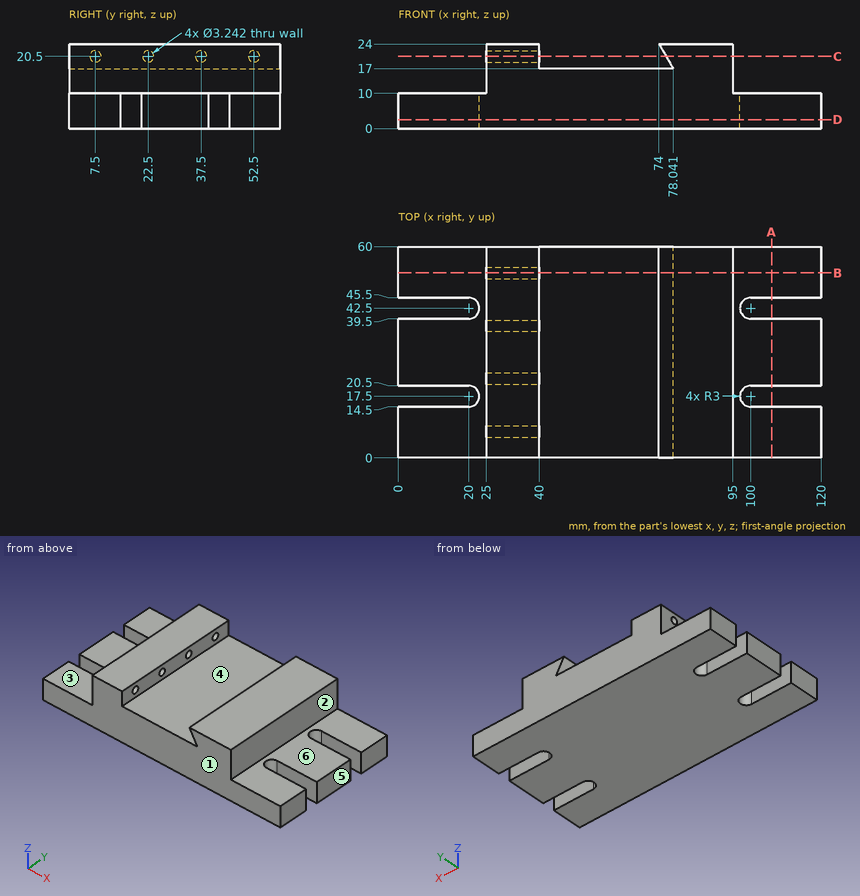
Geometry: see drawing. Coordinates: mm, zero at the bounding-box minimum. A direction names the side the tool comes from. Coordinates: 2 decimals unless noted, no trailing zeros. Order: outer loops, then holes, each group sorted by start corner. A loop starts at its lowest first (then second) coordinate and runs counter-clockwise, first axis right, second up. Notation, with made-up numbers: (-27, 75.25) - (2, 75.25) arc R21 ccw to (2, 102.25) - close; hole circle Ø3 at (63, 3). An arc over 180 degrees is marked (long way). Use one line per item in the form item = value.
1) Section A-A (x = 106). Return loops of the section in (y, z), then the cut area to 3 significant figures.
Solutions:
outline = (0, 0) - (14.5, 0) - (14.5, 10) - (0, 10) - close; (20.5, 0) - (39.5, 0) - (39.5, 10) - (20.5, 10) - close; (45.5, 0) - (60, 0) - (60, 10) - (45.5, 10) - close
area = 480 mm^2
2) Set-up query: the marked faces 1, 2 and 3. Return all of +Z, -Z, +X, -X, +Y, -Y with unobstructed straight access to the full face (end or side cutting, diameter ignored); none if empty.
Solutions:
face_1 = +Z, -Z, +X, -X, -Y
face_2 = +Z, +X, +Y, -Y
face_3 = +Z, -X, +Y, -Y
3) Ray query, L1, parallel to Y at x = 29.25, z = 20.5; L2, parallel to Z at x = 30.5, y = 7.5; L3, parallel to X at y = 9, z = 16.5. Return the intervals inside material, ascending.
Solutions:
L1 = 0 to 5.88, 9.12 to 20.88, 24.12 to 35.88, 39.12 to 50.88, 54.12 to 60
L2 = 0 to 18.88, 22.12 to 24
L3 = 25 to 95
4) Section D-D (z = 2.5). Return loops of the section in (x, y), then the cut area to 3 significant figures.
Solutions:
outline = (0, 0) - (120, 0) - (120, 14.5) - (100, 14.5) arc R3 cw to (100, 20.5) - (120, 20.5) - (120, 39.5) - (100, 39.5) arc R3 cw to (100, 45.5) - (120, 45.5) - (120, 60) - (0, 60) - (0, 45.5) - (20, 45.5) arc R3 cw to (20, 39.5) - (0, 39.5) - (0, 20.5) - (20, 20.5) arc R3 cw to (20, 14.5) - (0, 14.5) - close
area = 6,660 mm^2
5) Section B-B (y = 52.5). Return loops of the section in (x, z), then the cut area to 3 significant figures.
Solutions:
outline = (0, 0) - (120, 0) - (120, 10) - (95, 10) - (95, 24) - (74, 24) - (78.04, 17) - (40, 17) - (40, 18.88) - (25, 18.88) - (25, 10) - (0, 10) - close; (25, 22.12) - (40, 22.12) - (40, 24) - (25, 24) - close
area = 1,880 mm^2
6) Pin query (flat end, axial travel): pin 1 (7 mm diameter, centred on y = 23, z = 19.5, fed in from -X); pin 2 (1.9 mm diameter, centred on y = 37.5, z = 20.5, fed in from -X); pin 3 (5.5 mm diameter, centred on y = 38, z = 21, fed in from +X). Return the tip coordinate at first contact, or that it passes through.
Solutions:
pin_1 = 25
pin_2 = 75.47
pin_3 = 95
7) Section C-C (z = 20.5). Return loops of the section in (x, y), then the cut area to 3 significant figures.
Solutions:
outline = (25, 0) - (40, 0) - (40, 5.88) - (25, 5.88) - close; (25, 9.12) - (40, 9.12) - (40, 20.88) - (25, 20.88) - close; (25, 24.12) - (40, 24.12) - (40, 35.88) - (25, 35.88) - close; (25, 39.12) - (40, 39.12) - (40, 50.88) - (25, 50.88) - close; (25, 54.12) - (40, 54.12) - (40, 60) - (25, 60) - close; (76.02, 0) - (95, 0) - (95, 60) - (76.02, 60) - close
area = 1,840 mm^2
8) Mould query, pull axis X, two halves, no side actions, for the marked faces 4, 5 and 6. Classes: +X half, -X half, draft (parallel to the pull), parting line (faces both ways), or undercut.
Solutions:
face_4 = undercut
face_5 = +X half
face_6 = draft
